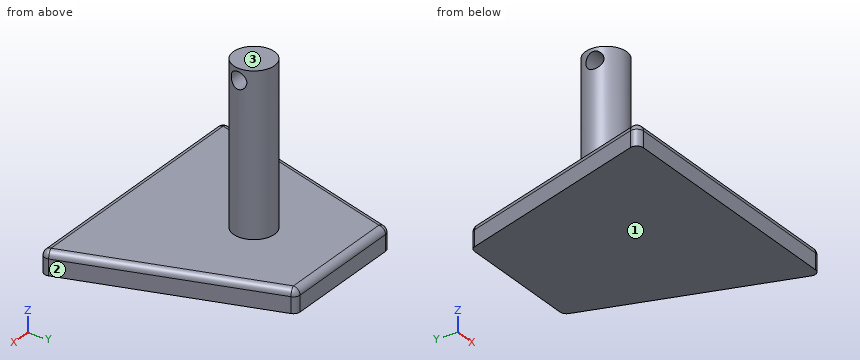
```python
from build123d import *

# Parameters (mm, degrees)
F0_W     = 200
F0_H     = 160
F1_DEPTH = 17
F3_DEPTH = 17.001
F4_R     = 5
F5_R     = 15.4974026332
F6_DEPTH = 120
F7_R     = 6.3299000504
F8_DEPTH = 41.6


with BuildPart() as f1:
    # F0 (on Top) → F1 (new body)
    with BuildSketch(Plane.XY):
        with Locations((5.6164655834, 14.2621519414)):
            Rectangle(F0_W, F0_H)
    extrude(amount=F1_DEPTH)

    # F2 (on face) → F3 (cut, through all)
    with BuildSketch(Plane.XY.offset(17)):
        Polygon((-94.3835344166, 94.2621519414), (-94.3835344166, -65.7378480586), (-44.3835344166, 94.2621519414), align=None)
        Polygon((55.6164655834, 94.2621519414), (105.6164655834, -65.7378480586), (105.6164655834, 94.2621519414), align=None)
    extrude(amount=-F3_DEPTH, mode=Mode.SUBTRACT)

    # F4
    f4_edges = [f1.edges().sort_by_distance(p)[0] for p in [
        (-94.383534, -65.737848, 8.5),
        (105.616466, -65.737848, 8.5),
        (55.616466, 94.262152, 8.5),
        (-44.383534, 94.262152, 8.5),
        (80.616466, 14.262152, 17),
        (5.616466, -65.737848, 17),
        (-69.383534, 14.262152, 17),
        (5.616466, 94.262152, 17),
    ]]
    fillet(f4_edges, radius=F4_R)

    # F5 (on face) → F6 (join)
    with BuildSketch(Plane.XY.offset(17)):
        with Locations((5.6164655834, 27.3357126862)):
            Circle(F5_R)
    extrude(amount=F6_DEPTH)

    # F7 (on Right) → F8 (cut, symmetric)
    with BuildSketch(Plane.YZ):
        with Locations((25.8725117892, 128.2121986151)):
            Circle(F7_R)
    extrude(amount=F8_DEPTH, both=True, mode=Mode.SUBTRACT)


solid = f1.part
```
Geometry: final body of the model. Coordinates: model frame, mm. Face numbers are marked on the shaded views. Round coordinates to 2 decimals unless told otherwise and drop trailing zeros. Write each loop counter-clockwise with the first axis right and the second up, starting at its lowest first coordinate (ties: lowest second). Pieces come first, ordered by that corner, then holes.
Item 1: Section query B-B (z = 49.5). Return loops of the section in (x, y).
Item 2: Section query A-A (x = 30.5). Return loops of the section in (y, z).
Item 3: Material intervals for L1, parallel to Z at x = 75.5, y = -54; L2, parallel to Y at x = 8, z = 40; L3, parallel to Y at x = -5, z = 105.5, sorted ascending.
Item 4: Pin query (flat end, axial travel): P1, Ø5, axis at x = 44, z = 17.5, coming from the -Y side; P2, Ø14.5, axis at y = 25.87, z = 128.21, coming from the -X side; P3, Ø10, axis at x = 69.5, y = -38.5, coming from the +Z side. Return the tip coordinate at first contact, or that it passes through.
Item 5: Mould query, pull axis Z, two halves, no side actions, for the marked faces 1, 2 and 3. Classes: +Z half, -Z half, draft (parallel to the pull), parting line (faces both ways), or undercut.
Completed:
1. outline: circle Ø30.99 at (5.62, 27.34)
2. outline: (-65.74, 0) - (94.26, 0) - (94.26, 12) arc R5 ccw to (89.26, 17) - (-60.74, 17) arc R5 ccw to (-65.74, 12) - close
3. L1: z = 0 to 17
3. L2: y = 12.02 to 42.65
3. L3: y = 16.05 to 38.63
4. P1: stops at y = -64.74
4. P2: stops at x = -9.88
4. P3: stops at z = 17
5. face 1: -Z half
5. face 2: draft
5. face 3: +Z half
